```python
from build123d import *

# Parameters (mm, degrees)
F0_R     = 36.775491
F0_R_2   = 33.454841
F0_R_3   = 3
F1_DEPTH = 2
F2_DEPTH = 3
F3_DEPTH = 1


with BuildPart() as f1:
    # F0 (on Top) → F1 (new body)
    with BuildSketch(Plane.XY):
        with Locations((37.5, 37.5)):
            Circle(F0_R)
        with Locations((37.5, 37.5)):
            Circle(F0_R_2, mode=Mode.SUBTRACT)
        with Locations((37.5, 37.5)):
            Circle(F0_R_2)
        with BuildLine():
            ThreePointArc((33.878023, 14.721462), (20.150811, 13.532255), (15.808449, 26.60874))
            Line((15.808449, 26.60874), (34.38191, 33.208317))
            Line((34.38191, 33.208317), (33.878023, 14.721462))
        make_face(mode=Mode.SUBTRACT)
        with BuildLine():
            Line((41.155146, 13.504525), (40.61809, 33.208317))
            Line((40.61809, 33.208317), (58.044424, 27.01634))
            ThreePointArc((58.044424, 27.01634), (54.933486, 13.593501), (41.155146, 13.504525))
        make_face(mode=Mode.SUBTRACT)
        with BuildLine():
            ThreePointArc((14.717071, 33.905749), (9.344126, 46.593618), (20.438738, 54.764306))
            Line((20.438738, 54.764306), (32.454824, 39.139277))
            Line((32.454824, 39.139277), (14.717071, 33.905749))
        make_face(mode=Mode.SUBTRACT)
        with Locations((37.5, 37.5)):
            Circle(F0_R_3, mode=Mode.SUBTRACT)
        with BuildLine():
            Line((61.450556, 33.561241), (42.545176, 39.139277))
            Line((42.545176, 39.139277), (53.819129, 53.79928))
            ThreePointArc((53.819129, 53.79928), (65.623675, 46.692716), (61.450556, 33.561241))
        make_face(mode=Mode.SUBTRACT)
        with BuildLine():
            Line((37.5, 42.804812), (27.041352, 58.057169))
            ThreePointArc((27.041352, 58.057169), (37.447901, 67.08791), (48.647111, 59.061188))
            Line((48.647111, 59.061188), (37.5, 42.804812))
        make_face(mode=Mode.SUBTRACT)
    extrude(amount=F1_DEPTH)

    # F0 (on Top) → F2 (join)
    with BuildSketch(Plane.XY):
        with Locations((37.5, 37.5)):
            Circle(F0_R)
        with Locations((37.5, 37.5)):
            Circle(F0_R_2, mode=Mode.SUBTRACT)
    extrude(amount=F2_DEPTH)

    # F0 (on Top) → F3 (join)
    with BuildSketch(Plane.XY):
        with BuildLine():
            Line((32.454824, 39.139277), (20.438738, 54.764306))
            ThreePointArc((20.438738, 54.764306), (9.344126, 46.593618), (14.717071, 33.905749))
            Line((14.717071, 33.905749), (32.454824, 39.139277))
        make_face()
        with BuildLine():
            ThreePointArc((48.647111, 59.061188), (37.447901, 67.08791), (27.041352, 58.057169))
            Line((27.041352, 58.057169), (37.5, 42.804812))
            Line((37.5, 42.804812), (48.647111, 59.061188))
        make_face()
        with BuildLine():
            Line((53.819129, 53.79928), (42.545176, 39.139277))
            Line((42.545176, 39.139277), (61.450556, 33.561241))
            ThreePointArc((61.450556, 33.561241), (65.623675, 46.692716), (53.819129, 53.79928))
        make_face()
        with BuildLine():
            Line((58.044424, 27.01634), (40.61809, 33.208317))
            Line((40.61809, 33.208317), (41.155146, 13.504525))
            ThreePointArc((41.155146, 13.504525), (54.933486, 13.593501), (58.044424, 27.01634))
        make_face()
        with BuildLine():
            Line((34.38191, 33.208317), (15.808449, 26.60874))
            ThreePointArc((15.808449, 26.60874), (20.150811, 13.532255), (33.878023, 14.721462))
            Line((33.878023, 14.721462), (34.38191, 33.208317))
        make_face()
    extrude(amount=F3_DEPTH)


solid = f1.part
```
Could you check a few things on this model? Use its own coordinates, in mm. A direction names the side the tool comes from. Round coordinates to 2 decimals unless told otherwise and drop trailing zeros. Order: outer loops, then holes, each group sorted by start corner. A loop starts at its lowest first (then second) coordinate and runs counter-clockwise, first axis right, second up. Notation, with made-up numbers: (-38.5, -24.75) -> (-2.5, -24.75) arc R31 ccw to (-2.5, 0.25) -> close; hole circle Ø7 at (36, 56.25). An arc over 180 degrees is marked (long way). One line per question, with ' | ' between items.
Q1. If I drill on line 1 (X direction, y = 38.5, z = 2.45); line 2 (Y direction, x = 37.5, z = 0.65); line 3 (Y direction, x = 37.5, z = 2.55), over which ranges is the centre line in solid material (lowest first)? Write a range as from..to.
Computed values:
line 1: 0.74..4.06, 70.94..74.26 | line 2: 0.72..34.5, 40.5..74.28 | line 3: 0.72..4.05, 70.95..74.28
Q2. If we section it at B-B on z = 1.5: Write out the boundary of the cut face in (x, y), plus the area to 3 significant figures.
Computed values:
outline: circle Ø73.55 at (37.5, 37.5); hole (14.72, 33.91) -> (32.45, 39.14) -> (20.44, 54.76) arc R11.12 ccw to start; hole (15.81, 26.61) arc R11.12 ccw to (33.88, 14.72) -> (34.38, 33.21) -> close; hole (27.04, 58.06) -> (37.5, 42.8) -> (48.65, 59.06) arc R11.12 ccw to start; hole circle Ø6 at (37.5, 37.5); hole (40.62, 33.21) -> (41.16, 13.5) arc R11.12 ccw to (58.04, 27.02) -> close; hole (42.55, 39.14) -> (61.45, 33.56) arc R11.12 ccw to (53.82, 53.8) -> close | area: 2,680 mm²
Q3. If we section it at C-C on y = 61: Write out the boundary of the cut face in (x, z), plus the area to 3 significant figures.
Computed values:
outline: (9.21, 0) -> (65.79, 0) -> (65.79, 3) -> (61.31, 3) -> (61.31, 2) -> (47.89, 2) -> (47.89, 1) -> (28.04, 1) -> (28.04, 2) -> (13.69, 2) -> (13.69, 3) -> (9.21, 3) -> close | area: 102 mm²
Q4. If we section it at A-A on y = 37.5: Write out the boundary of the cut face in (x, z).
Computed values:
outline: (0.72, 0) -> (34.5, 0) -> (34.5, 2) -> (26.9, 2) -> (26.9, 1) -> (10.81, 1) -> (10.81, 2) -> (4.05, 2) -> (4.05, 3) -> (0.72, 3) -> close; (40.5, 0) -> (74.28, 0) -> (74.28, 3) -> (70.95, 3) -> (70.95, 2) -> (65.01, 2) -> (65.01, 1) -> (48.1, 1) -> (48.1, 2) -> (40.5, 2) -> close
Q5. We'd pull the mould along Y, two halves only. Please class faces 1 (the face through (72.577, 48.546, 1.479)), 2 (the face through (24.965, 29.862, 1.493)), 3 (the face through (37, 30, 0)), 4 (the face through (49.209, 30.156, 1.493)): released by +Y, released by -Y, zero draft, split by the parting line, or undercut.
Computed values:
face 1: split by the parting line | face 2: undercut | face 3: zero draft | face 4: undercut
Q6. Which directions (+Z, -Z, +X, -X, +Y, -Y) give clear straight access to the entire face, cutting with the end or side of a thin tool? Please do faces 5 (the face through (50, 22, 1)), 6 (the face through (54, 8, 3)).
Computed values:
face 5: +Z | face 6: +Z, +X, -X, +Y, -Y
Q7. If we section it at D-D on y = 30: Write out the boundary of the cut face in (x, z), plus the area to 3 significant figures.
Computed values:
outline: (1.5, 0) -> (73.5, 0) -> (73.5, 3) -> (70.1, 3) -> (70.1, 2) -> (49.65, 2) -> (49.65, 1) -> (40.71, 1) -> (40.71, 2) -> (34.29, 2) -> (34.29, 1) -> (25.35, 1) -> (25.35, 2) -> (4.9, 2) -> (4.9, 3) -> (1.5, 3) -> close | area: 133 mm²
Q8. I'm going to push flat-ended pins straight in: pin 1 (10.5 mm diameter, centred on x = 18, y = 39.5, fed in from +Z); pin 2 (1 mm diameter, centred on y = 34, z = 2, fed in from +X); pin 3 (1 mm diameter, centred on y = 36.5, z = 0.5, fed in from -X). Where does each tip first touch, or does it pass through?
Computed values:
pin 1: z = 2 | pin 2: x = 74.15 | pin 3: x = 0.73
